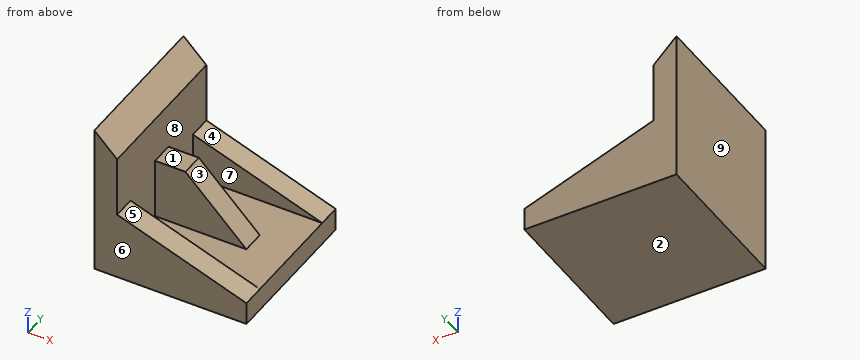
from build123d import *

# Parameters (mm, degrees)
F1_DEPTH = 127
F2_DEPTH = 19.05
F4_DEPTH = 38.1


# Not quite as in the source:
# - a pattern or mirror of a feature is missing from the dataset's text; its kind, count and spacing are read off the source's solid


with BuildPart() as f1:
    # F0 (on Front) → F1 (new body, symmetric)
    with BuildSketch(Plane.XZ):
        Polygon((0, 254), (0, 0), (254, 0), (254, 38.1), (190.5, 38.1), (38.1, 38.1), (38.1, 139.7), (38.1, 215.9), align=None)
    extrude(amount=F1_DEPTH, both=True)

    # F0 (on Front) → F2 (join, symmetric)
    with BuildSketch(Plane.XZ):
        Polygon((38.1, 38.1), (190.5, 38.1), (88.9, 139.7), (38.1, 139.7), align=None)
    extrude(amount=F2_DEPTH, both=True)

    # F3 (on face) → F4 (join)
    with BuildSketch(Plane.XZ.offset(127)):
        Polygon((254, 38.1), (38.1, 114.3), (38.1, 38.1), align=None)
    f4 = extrude(amount=-F4_DEPTH)

    # F4_copies: F4 across plane
    add(f4.mirror(Plane.ZX))


solid = f1.part
Source: CAD feature listing. Evaluate the final solid. Frame: model axes, mm. Face numbers are marked on the shaded views. A direction names the side the tool comes from. Round coordinates to 2 decimals unless told otherwise and drop trailing zeros. Loops run counter-clockwise (first coordinate to the right, second up) from the corner with the lowest first, then second, coordinate; pieces in that order, holes last. Notation, with made-up numbers: (71, 10) - (125, 10) arc R33 ccw to (125, 45) - close; hole circle Ø2 at (3, 51.25). An arc over 180 degrees is marked (long way). Write item = value, one per line. Start each with the question number.
(1) Section query A-A, the plane z = 87. Output: boundary loops of the cut face in (x, y).
(2) Ray query, line 1 along Y through (x, z) = (156, 55.5); line 2 along Z through (x, y) = (190.5, 33). Return the intervals inside material, ascending. Write a range as from..to.
(3) Section query B-B, the plane y = -7.5. Output: boundary loops of the cut face in (x, z).
(4) Section query C-C, the plane x = 58. Output: boundary loops of the cut face in (y, z), plus the area to 3 significant figures.
(5) Section query D-D, the plane y = -36.5. Output: boundary loops of the cut face in (x, z).
(6) Set-up query: the marked faces 1, 2, 3, 4 and 5. Return all of +Z, -Z, +X, -X, +Y, -Y with unobstructed straight access to the full face (end or side cutting, diameter ignored); none if empty.
(7) Pull-direction query (Y, two-part tool) for the marked faces 6, 7, 8 and 9; classes: +Y half, -Y half, draft (parallel to the pull), parting line (faces both ways), or undercut.
(8) Pin query (flat end, axial travel): pin 1 (1.5 mm diameter, centred on x = 45.5, y = -28.5, fed in from +Z); pin 2 (3 mm diameter, centred on y = -18, z = 55.5, fed in from +X); pin 3 (19 mm diameter, centred on x = 66, y = -0.5, fed in from +Z). Return the tip coordinate at first contact, or that it passes through.
Conclusion:
q1.outline = (0, -127) - (115.45, -127) - (115.45, -88.9) - (38.1, -88.9) - (38.1, -19.05) - (141.6, -19.05) - (141.6, 19.05) - (38.1, 19.05) - (38.1, 88.9) - (115.45, 88.9) - (115.45, 127) - (0, 127) - close
q2.line_1 = -127..-88.9, -19.05..19.05, 88.9..127
q2.line_2 = 0..38.1
q3.outline = (0, 0) - (254, 0) - (254, 38.1) - (190.5, 38.1) - (88.9, 139.7) - (38.1, 139.7) - (38.1, 215.9) - (0, 254) - close
q4.outline = (-127, 0) - (127, 0) - (127, 107.28) - (88.9, 107.28) - (88.9, 38.1) - (19.05, 38.1) - (19.05, 139.7) - (-19.05, 139.7) - (-19.05, 38.1) - (-88.9, 38.1) - (-88.9, 107.28) - (-127, 107.28) - close
q4.area = 18,800 mm2
q5.outline = (0, 0) - (254, 0) - (254, 38.1) - (38.1, 38.1) - (38.1, 215.9) - (0, 254) - close
q6.face_1 = +Z, +X, +Y, -Y
q6.face_2 = -Z, +X, -X, +Y, -Y
q6.face_3 = +Z, +X
q6.face_4 = +Z, +X, +Y
q6.face_5 = +Z, +X, -Y
q7.face_6 = -Y half
q7.face_7 = undercut
q7.face_8 = undercut
q7.face_9 = draft
q8.pin_1 = 38.1
q8.pin_2 = 174.6
q8.pin_3 = 139.7
